For this review, take the finished solid that the model builds, in its own axes (mm). Face numbers are marked on the shaded views. A direction names the side the tool comes from. Give positions to 0.01 mm unless a question says otherwise; leave off trailing zeros. Order: outer loops, then holes, each group sorted by start corner. A loop starts at its lowest first (then second) coordinate and runs counter-clockwise, first axis right, second up.
Item 1: For probe 1 along X at (y, z) = (14, 6.5); probe 2 along Y at (x, z) = (12, 4.5); probe 3 along Z at (x, y) = (-20.5, -6.5), list the stretches that pass through material, from the lowest coordinate up.
Item 2: Machinability: for the marked faces 5 and 6, which of the approach directions +Z, -Z, +X, -X, +Y, -Y give a long, thin tool a straight path to every point of the face, cutting with its end or side? Answer none if there is none.
Item 3: For P1, Ø6, axis at x = -9.5, z = -0.5, coming from the +Y side; P2, Ø4.5, axis at x = 6.5, z = 5.5, coming from the +Y side; P3, Ø12, axis at x = 26.5, y = 7, coming from the +Z side; P4, Ø6, axis at x = -8.5, y = 13.5, coming from the +Z side, all flat-tipped, find the tip position at first contact; note any pin that passes through.
Item 4: Consider section B-B (z = 2.5). Give the boundary of the cut face in (x, y).
Item 5: Consider section C-C (y = -26). Give the boundary of the cut face in (x, z).
Item 6: The part is to be moulded in two halves that separate along X. For the marked faces 1, 2, 3 and 4, say which applies: released by +X, released by -X, zero draft, split by the parting line, or undercut.
Item 7: Consider section A-A (x = 13). Give the boundary of the cut face in (y, z).
Item 8: Consider section D-D (z = -1.5). Give the boundary of the cut face in (x, y).
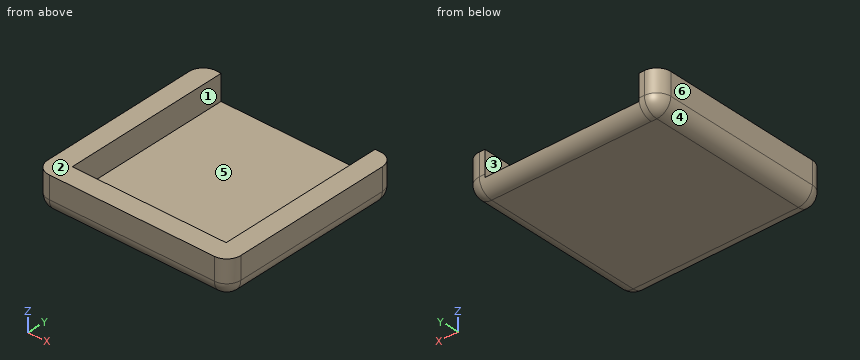
```python
from build123d import *

# Parameters (mm, degrees)
F1_DEPTH     = 9
F0_W         = 55
F0_H         = 60
F2_DEPTH     = 4
F3_T1_DEPTH  = 74.5
F3_T3_DEPTH  = 19.5
F3_T5_DEPTH  = 92
F3_T7_DEPTH  = 91.9996386864
F3_T9_DEPTH  = 93.9999999907
F4_T1_DEPTH  = 20.5
F4_T3_DEPTH  = 20.4993548139
F4_T8_DEPTH  = 5
F4_S13_W     = 5
F4_S13_H     = 5
F4_T14_DEPTH = 5
F4_S19_W     = 5
F4_S19_H     = 5
F4_T20_DEPTH = 5
F4_S25_W     = 5
F4_S25_H     = 5
F4_T26_DEPTH = 5


# Not quite as in the source:
# - a fillet or chamfer that OpenCascade refuses, or shapes differently, is made with other operations: its cross-section is extruded or revolved along the edge and cut away or added


with BuildPart() as f1:
    # F0 (on Top) → F1 (new body)
    with BuildSketch(Plane.XY):
        Polygon((27.5, 30), (27.5, -30), (-27.5, -30), (-27.5, 30), (-34.4999999907, 29.9996386864), (-34.4999999907, -37), (34.5, -37), (34.5, 30), align=None)
    extrude(amount=F1_DEPTH)

    # F0 (on Top) → F2 (join)
    with BuildSketch(Plane.XY):
        Polygon((27.5, 30), (27.5, -30), (-27.5, -30), (-27.5, 30), (-34.4999999907, 29.9996386864), (-34.4999999907, -37), (34.5, -37), (34.5, 30), align=None)
        Rectangle(F0_W, F0_H)
    extrude(amount=-F2_DEPTH)

    # F3: fillet of radius 5 on 5 edges, made by hand

    # F3_s2 → F3_t1 (cut)
    with BuildSketch(Plane.YZ.offset(-27.5)):
        with BuildLine():
            ThreePointArc((25, -4), (28.5355339059, -2.5355339059), (30, 1))
            Line((30, 1), (30, -4))
            Line((30, -4), (25, -4))
        make_face()
    extrude(amount=F3_T1_DEPTH, mode=Mode.SUBTRACT)

    # F3_s4 → F3_t3 (cut)
    with BuildSketch(Plane(origin=(-27.4984514401, -0.0014193662, 0), x_dir=(0, 0, 1), z_dir=(-0.9999999987, -5.16162e-05, 0))):
        with BuildLine():
            ThreePointArc((-4, 25.0014194062), (-2.5355339059, 28.5369533121), (1, 30.0014194062))
            Line((1, 30.0014194062), (-4, 30.0014194062))
            Line((-4, 30.0014194062), (-4, 25.0014194062))
        make_face()
    extrude(amount=F3_T3_DEPTH, mode=Mode.SUBTRACT)

    # F3_s6 → F3_t5 (cut)
    with BuildSketch(Plane.XZ.offset(-42.5)):
        with BuildLine():
            ThreePointArc((29.5, -4), (33.0355339059, -2.5355339059), (34.5, 1))
            Line((34.5, 1), (34.5, -4))
            Line((34.5, -4), (29.5, -4))
        make_face()
    extrude(amount=F3_T5_DEPTH, mode=Mode.SUBTRACT)

    # F3_s8 → F3_t7 (cut)
    with BuildSketch(Plane.XZ.offset(-42.4996386864)):
        with BuildLine():
            ThreePointArc((-34.4999999907, 1), (-33.0355338966, -2.5355339059), (-29.4999999907, -4))
            Line((-29.4999999907, -4), (-34.4999999907, -4))
            Line((-34.4999999907, -4), (-34.4999999907, 1))
        make_face()
    extrude(amount=F3_T7_DEPTH, mode=Mode.SUBTRACT)

    # F3_s10 → F3_t9 (cut)
    with BuildSketch(Plane.YZ.offset(-46.9999999907)):
        with BuildLine():
            ThreePointArc((-32, -4), (-35.5355339059, -2.5355339059), (-37, 1))
            Line((-37, 1), (-37, -4))
            Line((-37, -4), (-32, -4))
        make_face()
    extrude(amount=F3_T9_DEPTH, mode=Mode.SUBTRACT)

    # F4: fillet of radius 5 on 4 edges, made by hand

    # F4_s2 → F4_t1 (cut)
    with BuildSketch(Plane.XY.offset(1)):
        with BuildLine():
            ThreePointArc((-34.4999999907, -32), (-33.0355338966, -35.5355339059), (-29.4999999907, -37))
            Line((-29.4999999907, -37), (-34.4999999907, -37))
            Line((-34.4999999907, -37), (-34.4999999907, -32))
        make_face()
        with BuildLine():
            ThreePointArc((29.5, -37), (33.0355339059, -35.5355339059), (34.5, -32))
            Line((34.5, -32), (34.5, -37))
            Line((34.5, -37), (29.5, -37))
        make_face()
        with BuildLine():
            ThreePointArc((34.5, 25), (33.0355339059, 28.5355339059), (29.5, 30))
            Line((29.5, 30), (34.5, 30))
            Line((34.5, 30), (34.5, 25))
        make_face()
    extrude(amount=F4_T1_DEPTH, mode=Mode.SUBTRACT)

    # F4_s4 → F4_t3 (cut)
    with BuildSketch(Plane.XY.offset(1)):
        with BuildLine():
            ThreePointArc((-34.4999999907, 24.9998967609), (-33.0356251409, 28.5353394202), (-29.5002580718, 29.9998967542))
            Line((-29.5002580718, 29.9998967542), (-34.4999999907, 29.9996386864))
            Line((-34.4999999907, 29.9996386864), (-34.4999999907, 24.9998967609))
        make_face()
    extrude(amount=F4_T3_DEPTH, mode=Mode.SUBTRACT)


with BuildPart() as f4_tool6:
    # F4_s7 → F4_t8 (new body)
    with BuildSketch(Plane.XY.offset(1)):
        Polygon((-29.4999999907, 24.9998967609), (-34.4999999907, 24.9998967609), (-34.4999999907, 29.9996386864), (-29.5002580718, 29.9998967542), align=None)
    extrude(amount=-F4_T8_DEPTH)

    # F4_s9 → F4_t10 (revolve, cut)
    with BuildSketch(Plane(origin=(-29.4999999907, 24.9998967609, 1), x_dir=(0.70712503, -0.7070885319, 0), z_dir=(0.7070885319, 0.70712503, 0))):
        with BuildLine():
            ThreePointArc((0, -5), (5, 0), (0, 5))
            Line((0, 5), (0, -5))
        make_face()
    revolve(axis=Axis((-29.4999999907, 24.9998967609, 1), (0, 0, -1)), mode=Mode.SUBTRACT)


with BuildPart() as f1_1:
    add(f1.part)

    # F4_t5: cut F4_tool6
    add(f4_tool6.part, mode=Mode.SUBTRACT)


with BuildPart() as f4_tool12:
    # F4_s13 → F4_t14 (new body)
    with BuildSketch(Plane.YZ.offset(29.5)):
        with Locations((27.5, -1.5)):
            Rectangle(F4_S13_W, F4_S13_H)
    extrude(amount=F4_T14_DEPTH)

    # F4_s15 → F4_t16 (revolve, cut)
    with BuildSketch(Plane(origin=(29.5, 25, 1), x_dir=(0, -0.7071067812, 0.7071067812), z_dir=(0, 0.7071067812, 0.7071067812))):
        with BuildLine():
            ThreePointArc((0, -5), (5, 0), (0, 5))
            Line((0, 5), (0, -5))
        make_face()
    revolve(axis=Axis((29.5, 25, 1), (1, 0, 0)), mode=Mode.SUBTRACT)


with BuildPart() as f1_2:
    add(f1_1.part)

    # F4_t11: cut F4_tool12
    add(f4_tool12.part, mode=Mode.SUBTRACT)


with BuildPart() as f4_tool18:
    # F4_s19 → F4_t20 (new body)
    with BuildSketch(Plane.XZ.offset(32)):
        with Locations((32, -1.5)):
            Rectangle(F4_S19_W, F4_S19_H)
    extrude(amount=F4_T20_DEPTH)

    # F4_s21 → F4_t22 (revolve, cut)
    with BuildSketch(Plane(origin=(29.5, -32, 1), x_dir=(-0.7071067812, 0, 0.7071067812), z_dir=(0.7071067812, 0, 0.7071067812))):
        with BuildLine():
            ThreePointArc((0, -5), (5, 0), (0, 5))
            Line((0, 5), (0, -5))
        make_face()
    revolve(axis=Axis((29.5, -32, 1), (0, -1, 0)), mode=Mode.SUBTRACT)


with BuildPart() as f1_3:
    add(f1_2.part)

    # F4_t17: cut F4_tool18
    add(f4_tool18.part, mode=Mode.SUBTRACT)


with BuildPart() as f4_tool24:
    # F4_s25 → F4_t26 (new body)
    with BuildSketch(Plane.YZ.offset(-29.4999999907)):
        with Locations((-34.5, -1.5)):
            Rectangle(F4_S25_W, F4_S25_H)
    extrude(amount=-F4_T26_DEPTH)

    # F4_s27 → F4_t28 (revolve, cut)
    with BuildSketch(Plane(origin=(-29.4999999907, -32, 1), x_dir=(0, 0.7071067812, 0.7071067812), z_dir=(0, -0.7071067812, 0.7071067812))):
        with BuildLine():
            ThreePointArc((0, -5), (5, 0), (0, 5))
            Line((0, 5), (0, -5))
        make_face()
    revolve(axis=Axis((-29.4999999907, -32, 1), (-1, 0, 0)), mode=Mode.SUBTRACT)


with BuildPart() as f1_4:
    add(f1_3.part)

    # F4_t23: cut F4_tool24
    add(f4_tool24.part, mode=Mode.SUBTRACT)


solid = f1_4.part
```
Resolved:
1. probe 1: x = -34.5 to -27.5, 27.5 to 34.5
1. probe 2: y = -37 to -30
1. probe 3: z = -4 to 0
2. face 5: +Z, +Y
2. face 6: +Z, -Z, -X, +Y, -Y
3. P1: stops at y = 29.9
3. P2: stops at y = -30
3. P3: stops at z = 9
3. P4: stops at z = 0
4. outline: (-34.5, -32) arc R5 ccw to (-29.5, -37) - (29.5, -37) arc R5 ccw to (34.5, -32) - (34.5, 25) arc R5 ccw to (29.5, 30) - (27.5, 30) - (27.5, -30) - (-27.5, -30) - (-27.5, 30) - (-29.5, 30) arc R5 ccw to (-34.5, 25) - close
5. outline: (-34.5, 1) arc R5 ccw to (-29.5, -4) - (29.5, -4) arc R5 ccw to (34.5, 1) - (34.5, 9) - (27.5, 9) - (27.5, 0) - (-27.5, 0) - (-27.5, 9) - (-34.5, 9) - close
6. face 1: undercut
6. face 2: zero draft
6. face 3: undercut
6. face 4: released by -X
7. outline: (-37, 1) arc R5 ccw to (-32, -4) - (25, -4) arc R5 ccw to (29.9, 0) - (-30, 0) - (-30, 9) - (-37, 9) - close
8. outline: (-33.83, -32) arc R4.33 ccw to (-29.5, -36.33) - (29.5, -36.33) arc R4.33 ccw to (33.83, -32) - (33.83, 25) arc R4.33 ccw to (29.5, 29.33) - (-27.5, 29.33) - (-29.5, 29.33) arc R4.33 ccw to (-33.83, 25) - close
